Part model, mm, in its own coordinate system. A direction names the side the tool comes from. Coordinates: 2 decimals unless noted, no trailing zeros. Loops run counter-clockwise (first coordinate to the right, second up) from the corner with the lowest first, then second, coordinate; pieces in that order, holes last. Notation, with made-up numbers: (-34, -3.75) -> (12, -3.75) arc R13 cw to (12, 3.25) -> close; hole circle Ø9 at (15.5, -20). An arc over 180 degrees is marked (long way). Use one line per item in the form item = value. Start each with the question number.
(1) Pin check, flat tips, straight feed: P1, Ø1.2, axis at x = 14, z = 21, coming from the -Y side; P2, Ø2, axis at x = 13.5, z = 2.5, coming from the -Y side; P3, Ø1.2, axis at x = 13, y = -121, coming from the +Z side. Stop position of each tip, or through.
(2) 3-axis set-ups, long thin cutter, end or side, ignore diameter. For faces 1 (the flat face through (13, -115.724, 3)), 2 (the flat face through (13, -115.724, 41)), 3 (the flat face through (13, -119.724, 22)): which of +Z, -Z, +X, -X, +Y, -Y reach the whole face in a straight line?
(3) Band-saw the part on B-B on y = -98. Give the cut face in (x, z).
(4) Band-saw the part on C-C on z = 18.5. Give the cut face in (x, y), then the cut area to 3 significant figures.
(5) Mould opens along Y. For faces 4 (the flat face through (13, -123.834, 33)), 5 (the flat face through (13, -95.724, 3)), 6 (the flat face through (13, -103, 0.89)), 7 (the flat face through (13, -108, 5)) say: +Y half, -Y half, draft (parallel to the pull), parting line (faces both ways), or undercut.
(6) Drill centre lines: L1, parallel to Y at x = 15, z = 4; L2, parallel to Y at x = 12.35, z = 23.5; L3, parallel to Z at x = 13.9, y = -98.5. Where is each one in solid material? Low to high. Write a range as [from, to].
(7) Band-saw the part on A-A on x = 13. Give the cut face in (y, z).
```python
from build123d import *

# Parameters (mm, degrees)
BOSS_EXTRUDE1_DEPTH     = 4.11
PADDLE_MASTER_START     = 16.75
PADDLE_MASTER_OUTLINE_W = 4.11
PADDLE_MASTER_OUTLINE_H = 4.11
PADDLE_MASTER_DEPTH     = 10


# Read off the part's stored shape, not the designer's step: paddle_master
with BuildPart() as part:
    # motor_support_side-paddle_master<2> → Boss-Extrude1 (new body)
    with BuildSketch(Plane(origin=(15.26, -123.833512511, 38.5), x_dir=(0, 0, -1), z_dir=(1, 0, 0))):
        Polygon((33.5, 34.11), (0, 34.11), (-4.11, 34.11), (-4.11, 28.11), (0, 28.11), (0, 24.11), (-4.11, 24.11), (-4.11, 18.11), (0, 18.11), (0, 14.11), (-4.11, 14.11), (-4.11, 8.11), (0, 8.11), (0, 0), (33.5, 0), (33.5, 8.11), (37.61, 8.11), (37.61, 14.11), (33.5, 14.11), (33.5, 18.11), (37.61, 18.11), (37.61, 24.11), (33.5, 24.11), (33.5, 28.11), (37.61, 28.11), (37.61, 34.11), align=None)
    extrude(amount=-BOSS_EXTRUDE1_DEPTH)

    # paddle_master outline → paddle_master (cut)
    with BuildSketch(Plane.XY.offset(PADDLE_MASTER_START)):
        with Locations((13.205, -121.778512511)):
            Rectangle(PADDLE_MASTER_OUTLINE_W, PADDLE_MASTER_OUTLINE_H)
    extrude(amount=PADDLE_MASTER_DEPTH, mode=Mode.SUBTRACT)


solid = part.part
```
A:
q1.P1 = -119.72
q1.P2 = -115.72
q1.P3 = 38.5
q2.face_1 = -Z, +X, -X, -Y
q2.face_2 = +Z, +X, -X, -Y
q2.face_3 = +X, -X, -Y
q3.outline = (11.15, 5) -> (15.26, 5) -> (15.26, 38.5) -> (11.15, 38.5) -> close
q4.outline = (11.15, -119.72) -> (15.26, -119.72) -> (15.26, -89.72) -> (11.15, -89.72) -> close
q4.area = 123 mm²
q5.face_4 = -Y half
q5.face_5 = undercut
q5.face_6 = draft
q5.face_7 = undercut
q6.L1 = [-115.72, -109.72], [-105.72, -99.72], [-95.72, -89.72]
q6.L2 = [-119.72, -89.72]
q6.L3 = [5, 38.5]
q7.outline = (-123.83, 5) -> (-115.72, 5) -> (-115.72, 0.89) -> (-109.72, 0.89) -> (-109.72, 5) -> (-105.72, 5) -> (-105.72, 0.89) -> (-99.72, 0.89) -> (-99.72, 5) -> (-95.72, 5) -> (-95.72, 0.89) -> (-89.72, 0.89) -> (-89.72, 42.61) -> (-95.72, 42.61) -> (-95.72, 38.5) -> (-99.72, 38.5) -> (-99.72, 42.61) -> (-105.72, 42.61) -> (-105.72, 38.5) -> (-109.72, 38.5) -> (-109.72, 42.61) -> (-115.72, 42.61) -> (-115.72, 38.5) -> (-123.83, 38.5) -> (-123.83, 26.75) -> (-119.72, 26.75) -> (-119.72, 16.75) -> (-123.83, 16.75) -> close
